The model under review builds one solid part; all positions refer to its coordinate system, in mm. A direction names the side the tool comes from. Round coordinates to 2 decimals unless told otherwise and drop trailing zeros. Write each loop counter-clockwise with the first axis right and the second up, starting at its lowest first coordinate (ties: lowest second). Pieces come first, ordered by that corner, then holes. Notation, with made-up numbers: M 2,87.5 L 57,87.5 A24 cw 57,97.5 Z; hole C 84,81 d9. An arc over 180 degrees is marked long. One line per item, written item: value. Start each with the question number.
1) Mouldability with a two-part tool opening along Z and no side actions: class faces 6 (the face through (14.985, -6.261, 0.66)), 7 (the face through (-1, -98, 100)), 8 (the face through (26.75, -29.58, 93.74)) as +Z half, -Z half, draft (parallel to the pull), parting line (faces both ways), or undercut.
2) Take a section at C-C, the plane x = 0. Write out the cut boundary in (y, z), and give its area (3 significant figures).
3) Take a section at D-D, the plane z = 43.5. Write out the cut boundary in (x, y).
4) Tool access review of faces 1 (the face through (-54, -158, -87.3)), 2 (the face through (-93.739, -56.698, 54.787)), 3 (the face through (-96.38, -99.93, 96.18)), 4 (the face through (-41.412, -116.865, 93.739)), 5 (the face through (-14.985, -191.198, 0.66)): name each direction out of +Z, -Z, +X, -X, +Y, -Y from which nothing blocks a thin tool from reaching the whole face with its end or side.
5) Take a section at A-A, the plane z = 0. Write out the cut boundary in (x, y), and give its area (3 significant figures).
6) Wall thickness on probe 1 along X at (y, z) = (-44.5, 40); probe 2 along Z at (x, y) = (44.5, -122.5); probe 3 along X at (y, z) = (-28.5, -45.5): over which ranges is each line inside the solid? List them lowest first.
7) For P1, Ø18, axis at x = 0, z = 0, coming from the -Y side; P2, Ø9, axis at y = -47, z = 54.5, coming from the -X side; P3, Ø15, axis at x = -50.5, z = 49.5, coming from the +Y side, all flat-tipped, find the tip position at first contact; note any pin that passes through.
from build123d import *

# Parameters (mm, degrees)
F0_W      = 200
F0_H      = 200
F1_DEPTH  = 197.4596
F2_R      = 12.7
F3_R      = 15
F4_DEPTH  = 12.7
F6_R      = 15
F7_DEPTH  = 12.7
F5_R      = 15
F8_DEPTH  = 12.7
F9_R      = 15
F10_DEPTH = 12.7
F11_R     = 15
F12_DEPTH = 12.7
F13_R     = 15
F14_DEPTH = 12.7


# Not quite as in the source:
# - a feature names something its author has since deleted; it is built from what else it names


with BuildPart() as f1:
    # F0 (on Front) → F1 (new body)
    with BuildSketch(Plane.XZ):
        Rectangle(F0_W, F0_H)
    extrude(amount=F1_DEPTH)

    # F2
    f2_edges = [f1.edges().sort_by_distance(p)[0] for p in [
        (100, -98.7298, -100),
        (100, -98.7298, 100),
        (100, 0, 0),
        (100, -197.4596, 0),
        (-100, -98.7298, 100),
        (0, 0, 100),
        (0, -197.4596, 100),
        (0, 0, -100),
        (-100, 0, 0),
        (-100, -98.7298, -100),
        (0, -197.4596, -100),
        (-100, -197.4596, 0),
    ]]
    fillet(f2_edges, radius=F2_R)

    # F3 (on face) → F4 (cut)
    with BuildSketch(Plane.XZ.offset(197.4596)):
        Circle(F3_R)
    extrude(amount=-F4_DEPTH, mode=Mode.SUBTRACT)

    # F6 (on face) → F7 (cut)
    with BuildSketch(Plane(origin=(0, 0, 0), x_dir=(-1, 0, 0), z_dir=(0, 1, 0))):
        with Locations((54.645486176, 53.4084625542)):
            Circle(F6_R)
        Circle(F6_R)
        with Locations((-55.5655397475, -50.3540486097)):
            Circle(F6_R)
    extrude(amount=-F7_DEPTH, mode=Mode.SUBTRACT)

    # F5 (on face) → F8 (cut)
    with BuildSketch(Plane.YZ.offset(100)):
        with Locations((-132.281050086, -34.5258712769)):
            Circle(F5_R)
        with Locations((-54.3126091361, 48.1324009597)):
            Circle(F5_R)
    extrude(amount=-F8_DEPTH, mode=Mode.SUBTRACT)

    # F9 (on face) → F10 (cut)
    with BuildSketch(Plane(origin=(-100, 0, 0), x_dir=(0, -1, 0), z_dir=(-1, 0, 0))):
        with Locations((42.3903614283, 50.2816922963)):
            Circle(F9_R)
        with Locations((39.9255715311, -43.3802828193)):
            Circle(F9_R)
        with Locations((148.3762711287, 55.2112646401)):
            Circle(F9_R)
        with Locations((153.7988185883, -42.8873226047)):
            Circle(F9_R)
    extrude(amount=-F10_DEPTH, mode=Mode.SUBTRACT)

    # F11 (on face) → F12 (cut)
    with BuildSketch(Plane(origin=(0, 0, -100), x_dir=(1, 0, 0), z_dir=(0, 0, -1))):
        with Locations((0, 105.1476597786)):
            Circle(F11_R)
        with Locations((53.2865412533, 56.5827190876)):
            Circle(F11_R)
        with Locations((-45.8668917418, 53.8846664131)):
            Circle(F11_R)
        with Locations((-53.9610497653, 157.759681344)):
            Circle(F11_R)
        with Locations((59.3571513891, 154.3871164322)):
            Circle(F11_R)
    extrude(amount=-F12_DEPTH, mode=Mode.SUBTRACT)

    # F13 (on face) → F14 (cut)
    with BuildSketch(Plane.XY.offset(100)):
        with Locations((-39.4590161741, -39.7198908031)):
            Circle(F13_R)
        with Locations((37.8009901579, -39.7198908031)):
            Circle(F13_R)
        with Locations((-39.4590161741, -82.2142139077)):
            Circle(F13_R)
        with Locations((34.062910825, -85.5867788196)):
            Circle(F13_R)
        with Locations((-39.4590161741, -131.7378137109)):
            Circle(F13_R)
        with Locations((35.4119352996, -132.8026950359)):
            Circle(F13_R)
    extrude(amount=-F14_DEPTH, mode=Mode.SUBTRACT)


solid = f1.part
Checked values:
1. face 6: undercut
1. face 7: +Z half
1. face 8: draft
2. outline: M -197.46,-87.3 A12.7 ccw -184.76,-100 L -120.15,-100 L -120.15,-87.3 L -90.15,-87.3 L -90.15,-100 L -12.7,-100 A12.7 ccw 0,-87.3 L 0,-15 L -12.7,-15 L -12.7,15 L 0,15 L 0,87.3 A12.7 ccw -12.7,100 L -184.76,100 A12.7 ccw -197.46,87.3 L -197.46,15 L -184.76,15 L -184.76,-15 L -197.46,-15 Z
2. area: 38,200 mm2
3. outline: M -100,-184.76 A12.7 ccw -87.3,-197.46 L 87.3,-197.46 A12.7 ccw 100,-184.76 L 100,-68.58 L 87.3,-68.58 L 87.3,-40.05 L 100,-40.05 L 100,-12.7 A12.7 ccw 87.3,0 L -43.38,0 L -43.38,-12.7 L -65.91,-12.7 L -65.91,0 L -87.3,0 A12.7 ccw -100,-12.7 L -100,-29.01 L -87.3,-29.01 L -87.3,-55.77 L -100,-55.77 L -100,-139 L -87.3,-139 L -87.3,-157.75 L -100,-157.75 Z
4. face 1: -Z
4. face 2: -X
4. face 3: +Z, -X, +Y, -Y
4. face 4: +Z
4. face 5: -Y
5. outline: M -100,-184.76 A12.7 ccw -87.3,-197.46 L -15,-197.46 L -15,-184.76 L 15,-184.76 L 15,-197.46 L 87.3,-197.46 A12.7 ccw 100,-184.76 L 100,-12.7 A12.7 ccw 87.3,0 L 15,0 L 15,-12.7 L -15,-12.7 L -15,0 L -87.3,0 A12.7 ccw -100,-12.7 Z
5. area: 38,600 mm2
6. probe 1: x = -87.3 to 87.3
6. probe 2: z = -100 to 87.3
6. probe 3: x = -87.3 to 100
7. P1: stops at y = -184.76
7. P2: stops at x = -87.3
7. P3: stops at y = -12.7
